from build123d import *

# Parameters (mm, degrees)
SKETCH1_R           = 7.5
SKETCH1_R_2         = 3.5
BOSS_EXTRUDE1_DEPTH = 7
SKETCH2_R           = 32.5
BOSS_EXTRUDE2_DEPTH = 208
BOSS_EXTRUDE3_START = 3
SKETCH3_R           = 23.5
SKETCH3_R_2         = 7.5
BOSS_EXTRUDE3_DEPTH = 3


with BuildPart() as part:
    # Sketch1 → Boss-Extrude1 (new body)
    with BuildSketch(Plane.XY):
        with BuildLine():
            Line((-27, -34), (27, -34))
            ThreePointArc((27, -34), (31.949747468, -31.949747468), (34, -27))
            Line((34, -27), (34, 27))
            ThreePointArc((34, 27), (31.949747468, 31.949747468), (27, 34))
            Line((27, 34), (-27, 34))
            ThreePointArc((-27, 34), (-31.949747468, 31.949747468), (-34, 27))
            Line((-34, 27), (-34, -27))
            ThreePointArc((-34, -27), (-31.949747468, -31.949747468), (-27, -34))
        make_face()
        Circle(SKETCH1_R, mode=Mode.SUBTRACT)
        with Locations((27.577164466, 27.577164466)):
            Circle(SKETCH1_R_2, mode=Mode.SUBTRACT)
        with Locations((-27.577164466, 27.577164466)):
            Circle(SKETCH1_R_2, mode=Mode.SUBTRACT)
        with Locations((-27.577164466, -27.577164466)):
            Circle(SKETCH1_R_2, mode=Mode.SUBTRACT)
        with Locations((27.577164466, -27.577164466)):
            Circle(SKETCH1_R_2, mode=Mode.SUBTRACT)
    extrude(amount=-BOSS_EXTRUDE1_DEPTH)

    # Sketch2 → Boss-Extrude2 (add)
    with BuildSketch(Plane(origin=(0, 0, -7), x_dir=(-1, 0, 0), z_dir=(0, 0, -1))):
        with Locations(Location((0, 0, 0), (0, 0, 180))):
            Circle(SKETCH2_R)
    extrude(amount=BOSS_EXTRUDE2_DEPTH)

    # Sketch3 → Boss-Extrude3 (add)
    with BuildSketch(Plane.XY.offset(BOSS_EXTRUDE3_START)):
        with Locations(Location((0, 0, 0), (0, 0, 180))):
            Circle(SKETCH3_R)
        Circle(SKETCH3_R_2, mode=Mode.SUBTRACT)
    extrude(amount=-BOSS_EXTRUDE3_DEPTH)


solid = part.part
Verification items for the finished model (mm, model axes). A direction names the side the tool comes from. Coordinates: 2 decimals unless noted, no trailing zeros. Order: outer loops, then holes, each group sorted by start corner. A loop starts at its lowest first (then second) coordinate and runs counter-clockwise, first axis right, second up. Notation, with made-up numbers: M 63,15.25 L 74,15.25 A24 cw 74,33.25 Z; hole C -27,10.25 d6. An arc over 180 degrees is marked long. Write each question's results on one line, items separated by ' | '.
1) Scan lines: line 1 along Z through (x, y) = (2.5, -27.5); line 2 along Y through (x, z) = (-9.5, -79); line 3 along Y through (x, z) = (15.5, -107). Record each from-to range of solid material in increasing order. Write a range as [from, to].
Solved:
line 1: z = [-215, 0] | line 2: y = [-31.08, 31.08] | line 3: y = [-28.57, 28.57]
2) Gauge pin test, flat ends, axial feed: pin 1 Ø6.5 at (x, y) = (27.58, 27.58) entering from +Z; pin 2 Ø11 at (x, y) = (-27.58, 27.58) entering from +Z; pin 3 Ø6 at (x, z) = (0.5, -43.5) entering from -Y; pin 4 Ø1 at (y, z) = (27, -95) entering from -X. Record the tip position at first contact, or that the pin passes through.
Solved:
pin 1: passes through | pin 2: stops at z = 0 | pin 3: stops at y = -32.5 | pin 4: stops at x = -18.81
3) Section check D-D on z = -197.5. Record the cut outline in (x, y), plus the area to 3 significant figures.
Solved:
outline: C 0,0 d65 | area: 3,320 mm²
4) Section check C-C on x = -29. Record the cut outline in (y, z).
Solved:
outline: M -33.71,-7 L -30.77,-7 L -30.77,0 L -33.71,0 Z; M -24.38,-7 L -14.67,-7 L -14.67,-215 L 14.67,-215 L 14.67,-7 L 24.38,-7 L 24.38,0 L -24.38,0 Z; M 30.77,-7 L 33.71,-7 L 33.71,0 L 30.77,0 Z
5) Release check for a two-part mould opening along X. For faces 4 (the face through (12.4, 30.4, -7)), 5 (the face through (-34, 0, -3)), 6 (the face through (32, 31.9, -3.5)), 7 (the face through (-24.24, 28.63, -3.45)) record: pulls with the +X half, pulls with the -X half, needs draft (parallel to the pull), parting line crosses it, or undercut.
Solved:
face 4: needs draft | face 5: pulls with the -X half | face 6: pulls with the +X half | face 7: undercut
6) Section check A-A on x = 0. Record the cut outline in (y, z), plus the area to 3 significant figures.
Solved:
outline: M -34,-7 L -32.5,-7 L -32.5,-215 L 32.5,-215 L 32.5,-7 L 34,-7 L 34,0 L 23.5,0 L 23.5,3 L 7.5,3 L 7.5,-7 L -7.5,-7 L -7.5,3 L -23.5,3 L -23.5,0 L -34,0 Z | area: 14,000 mm²
7) Access from +Z, -Z, +X, -X, +Y, -Y to the whole of each face (thin tool, end or side, straight path). Record for faces 1 (the face through (-7.493, 0.33, -1.93)), 2 (the face through (31, -9.76, -109.54)), 3 (the face through (0, -34, -3)).
Solved:
face 1: +Z | face 2: -Z | face 3: +Z, -Z, +X, -X, -Y
